For this review, take the finished solid that the model builds, in its own axes (mm). Give positions to 0.01 mm unless a question says otherwise; leave off trailing zeros. Order: outer loops, then holes, each group sorted by start corner. A loop starts at its lowest first (then second) coordinate and runs counter-clockwise, first axis right, second up. Notation, with made-up numbers: (37, 39) -> (84, 39) arc R20 cw to (84, 51) -> close; hole circle Ø7 at (37.25, -33). An arc over 180 degrees is marked (long way). Return JSON: item names as keys, results as strings. Group by question number.
1) Add section A-A (y = -86.2). Give the boundary of the cut face in (x, z) (1 decimal), then the cut area to 3 significant figures.
2) To check wall thickness, follow line 1 along Y through (x, z) = (0, 0.7); line 2 along X through (y, z) = (-70, 0.7); line 3 along X through (y, z) = (68, 1.3). State the ranges of each line that lie inside material, in increasing order.
3) Add section D-D (y = 0). Give the boundary of the cut face in (x, z) (3 decimals).
4) Add section B-B (x = 36.5). Give the boundary of the cut face in (y, z) (3 decimals), then the cut area to 3 significant figures.
5) Insertion check: P1, Ø8, axis at x = -81.98, y = 26.64, coming from the +Z side; P2, Ø4.5, axis at x = 81.98, y = -26.64, coming from the -Z side; P3, Ø1.5, axis at y = 69, z = 2.5, coming from the +X side; P4, Ø6.5, axis at x = 0, y = 86.2, coming from the +Z side. Each pin has a flat end and moves straight along its axis. Give the tip position at first contact, or say it passes through.
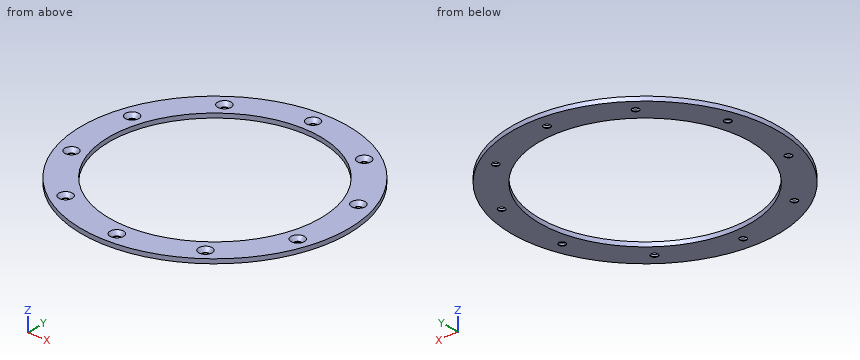
Autodesk Inventor part; units mm, degrees
ref_plane "YZ Plane" through (0, 0, 0) normal (1, 0, 0) x (0, 1, 0)
ref_plane "XZ Plane" through (0, 0, 0) normal (0, 1, 0) x (-1, 0, 0)
ref_plane "XY Plane" through (0, 0, 0) normal (0, 0, 1) x (1, 0, 0)
sketch "Sketch1" plane through (0, 0, 0) normal (0, 0, 1) x (1, 0, 0)
  circle A0 centre (0, 0) radius 76.2
  circle A1 centre (0, 0) radius 96.2
  dimension "d0" = 152.4
  dimension "d1" = 20
extrude "Extrusion1" add sketch "Sketch1" along normal blind 3.175
sketch "Sketch2" plane through (0, 0, 3.175) normal (0, 0, 1) x (1, 0, 0)
  circle A0 centre (0, 0) radius 76.2
  circle A1 centre (0, 0) radius 96.2
  circle A2 centre (0, 0) radius 76.2
  line L0 (0, 76.2) -> (0, 96.2)
  point P0 (0, 86.2)
  point P1 (0, 86.2)
hole "Hole1" at (0, 86.2, 3.175) direction (0, 0, -1) diameter 4.978 depth 8 tip angle 118 countersink diameter 9.779 countersink angle 82
pattern_circular "Circular Pattern1" count 10 over 360 about axis through (0, 0, 0) along (0, 0, 1) of "Hole1"
properties part number "1134_RU O Ring Cap_V1" material "Aluminum 6061"
Evaluation:
{
 "1": {"outline": "(-42.7, 0) -> (-2.5, 0) -> (-2.5, 0.4) -> (-4.9, 3.2) -> (-42.7, 3.2) -> close; (2.5, 0) -> (42.7, 0) -> (42.7, 3.2) -> (4.9, 3.2) -> (2.5, 0.4) -> close", "area": "249 mm^2"},
 "2": {"line 1": "-96.2 to -88.94, -83.46 to -76.2, 76.2 to 83.46, 88.94 to 96.2", "line 2": "-65.99 to -53.39, -47.94 to -30.11, 30.11 to 47.94, 53.39 to 65.99", "line 3": "-68.05 to -53.43, -47.91 to -34.39, 34.39 to 47.91, 53.43 to 68.05"},
 "3": {"outline": "(-96.2, 0) -> (-76.2, 0) -> (-76.2, 3.175) -> (-96.2, 3.175) -> close; (76.2, 0) -> (96.2, 0) -> (96.2, 3.175) -> (76.2, 3.175) -> close"},
 "4": {"outline": "(-89.007, 0) -> (-66.889, 0) -> (-66.889, 3.175) -> (-89.007, 3.175) -> close; (66.889, 0) -> (89.007, 0) -> (89.007, 3.175) -> (66.889, 3.175) -> close", "area": "140 mm^2"},
 "5": {"P1": "z = 2.16", "P2": "through", "P3": "x = 67.8", "P4": "z = 1.29"}
}
